Geometry: see drawing. Coordinates: mm, zero at the bounding-box minimum. Give positions to 0.01 mm unless a question says otherwise; leave off trailing zeros. Write each loop counter-clockwise with the first axis right and the second up, starting at its lowest first coordinate (ties: lowest second). Pieces come first, ordered by that corner, then holes. Notation, with made-up numbers: M 8,87.5 L 14,87.5 A17 ccw 14,91.5 Z; hole C 87.25,52.5 d9. An arc over 180 degrees is marked long. Use a Markdown table: item, result. Add a question column.
1) Line query: line 1 (Y direction, x = 2, z = 0.8); line 2 (X direction, y = 5.25, z = 0.8) (1 decimal); line 3 (Y direction, x = 1.6, z = 1.15). Output: solid intervals per line, ascending.
2) Section A-A on x = 2. Return the cut outline in (y, z).
3) Draft query along Y for the marked faces 1, 2, 3 and 4. Return one class per face: +Y half, -Y half, draft (parallel to the pull), parting line (faces both ways), or undercut.
4) Section C-C on x = 2.65. Return the cut outline in (y, z).
5) Section B-B on z = 0.45. Return the cut outline in (x, y).
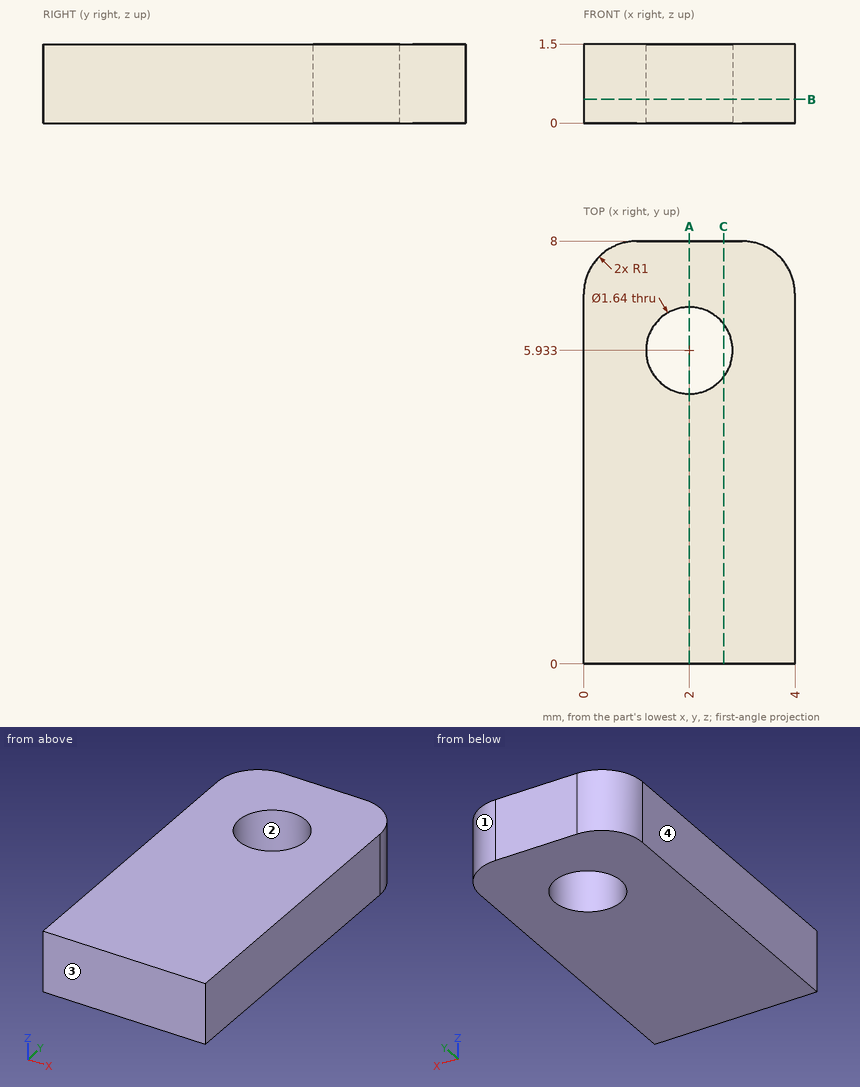
Found:
| question | item | result |
|---|---|---|
| 1 | line 1 | 0 to 5.11, 6.75 to 8 |
| 1 | line 2 | 0 to 1.5, 2.5 to 4 |
| 1 | line 3 | 0 to 5.22, 6.65 to 8 |
| 2 | outline | M 0,0 L 5.11,0 L 5.11,1.5 L 0,1.5 Z; M 6.75,0 L 8,0 L 8,1.5 L 6.75,1.5 Z |
| 3 | face 1 | +Y half |
| 3 | face 2 | undercut |
| 3 | face 3 | -Y half |
| 3 | face 4 | draft |
| 4 | outline | M 0,0 L 5.43,0 L 5.43,1.5 L 0,1.5 Z; M 6.43,0 L 8,0 L 8,1.5 L 6.43,1.5 Z |
| 5 | outline | M 0,0 L 4,0 L 4,7 A1 ccw 3,8 L 1,8 A1 ccw 0,7 Z; hole C 2,5.93 d1.64 |
